from build123d import *

# Parameters (mm, degrees)
SKETCH2_W           = 12.7
SKETCH2_H           = 6.35
SKETCH2_R           = 4
BOSS_EXTRUDE1_DEPTH = 6.35


with BuildPart() as part:
    # Sketch2 → Boss-Extrude1 (new body)
    # profile 1 of 3: a face of its own
    with BuildSketch(Plane.XY):
        with Locations((-16.409901661, -28.575)):
            Rectangle(SKETCH2_W, SKETCH2_H)
    # profile 2 of 3: a face of its own
    with BuildSketch(Plane.XY):
        with BuildLine():
            Line((22.759901661, -25.4), (11.934096284, 4.34365582))
            ThreePointArc((11.934096284, 4.34365582), (0, 12.7), (-11.934096284, 4.34365582))
            Line((-11.934096284, 4.34365582), (-22.759901661, -25.4))
            Line((-22.759901661, -25.4), (22.759901661, -25.4))
        make_face()
        Circle(SKETCH2_R, mode=Mode.SUBTRACT)
    # profile 3 of 3: a face of its own
    with BuildSketch(Plane.XY):
        with Locations((16.409901661, -28.575)):
            Rectangle(SKETCH2_W, SKETCH2_H)
    extrude(amount=BOSS_EXTRUDE1_DEPTH)


solid = part.part
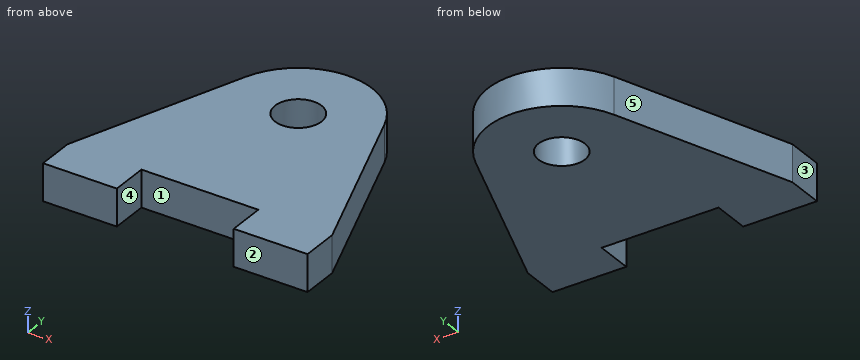
Source: CAD feature listing. Evaluate the final solid. Frame: model axes, mm. Face numbers are marked on the shaded views. A direction names the side the tool comes from. Coordinates: 2 decimals unless noted, no trailing zeros. Write each loop counter-clockwise with the first axis right and the second up, starting at its lowest first coordinate (ties: lowest second). Pieces come first, ordered by that corner, then holes. Notation, with made-up numbers: M 68,7.25 L 90,7.25 A16 ccw 90,28.25 Z; hole C 40,60.25 d10. An arc over 180 degrees is marked long. Use a Markdown table: item, result.
1) Section A-A, the plane y = -27. Output: boundary loops of the cut face in (x, z).
Conclusion:
| item | result |
|---|---|
| outline | M -22.76,0 L -10.06,0 L -10.06,6.35 L -22.76,6.35 Z; M 10.06,0 L 22.76,0 L 22.76,6.35 L 10.06,6.35 Z |
2) Reachability of the marked faces 4 and 5 from +Z, -Z, +X, -X, +Y, -Y: full face, straight path, thin tool, end or side. Return the list, or none.
Conclusion:
| item | result |
|---|---|
| face 4 | +Z, -Z, -Y |
| face 5 | +Z, -Z, -X, +Y |
3) Section B-B, the plane x = 0. Output: boundary loops of the cut face in (y, z).
Conclusion:
| item | result |
|---|---|
| outline | M -25.4,0 L -4,0 L -4,6.35 L -25.4,6.35 Z; M 4,0 L 12.7,0 L 12.7,6.35 L 4,6.35 Z |
4) Mould query, pull axis X, two halves, no side actions, for the marked faces 1, 2 and 3. Classes: pulls with the +X half, pulls with the -X half, needs draft (parallel to the pull), parting line crosses it, or undercut.
Conclusion:
| item | result |
|---|---|
| face 1 | undercut |
| face 2 | needs draft |
| face 3 | pulls with the -X half |
5) Section C-C, the plane z = 2.75. Output: boundary loops of the cut face in (x, y).
Conclusion:
| item | result |
|---|---|
| outline | M -22.76,-31.75 L -10.06,-31.75 L -10.06,-25.4 L 10.06,-25.4 L 10.06,-31.75 L 22.76,-31.75 L 22.76,-25.4 L 11.93,4.34 A12.7 ccw -11.93,4.34 L -22.76,-25.4 Z; hole C 0,0 d8 |
6) Ray query, L1, parallel to Y at x = 11, z = 3.5; L2, parallel to Y at x = -2.5, z = 4.5; L3, parallel to X at y = -0.5, z = 1.25. Return the intervals inside material, ascending.
Conclusion:
| item | result |
|---|---|
| L1 | y = -31.75 to 6.35 |
| L2 | y = -25.4 to -3.12, 3.12 to 12.45 |
| L3 | x = -13.7 to -3.97, 3.97 to 13.7 |
7) Section D-D, the plane x = 17. Output: boundary loops of the cut face in (y, z).
Conclusion:
| item | result |
|---|---|
| outline | M -31.75,0 L -9.57,0 L -9.57,6.35 L -31.75,6.35 Z |
8) First-contact query: pin 1 Ø2 at (y, z) = (7, 1) entering from -X; pin 2 Ø1.5 at (y, z) = (-1.5, 2) entering from +X; pin 3 Ø2 at (x, z) = (-7.5, 4) entering from +Y. Flat tips, straight axial feed; report the tip coordinate or a pass-through.
Conclusion:
| item | result |
|---|---|
| pin 1 | stops at x = -11.19 |
| pin 2 | stops at x = 14.33 |
| pin 3 | stops at y = 10.91 |
